from build123d import *

# Parameters (mm, degrees)
SKETCH_1_R      = 4
SKETCH_1_R_2    = 1.55
EXTRUDE_1_DEPTH = 4
SKETCH_2_R      = 10
SKETCH_2_R_2    = 1.55
EXTRUDE_2_DEPTH = 3


with BuildPart() as part:
    # 草图1 → 凸台-拉伸1 (new body)
    with BuildSketch(Plane(origin=(0, 0, 0), x_dir=(1, 0, 0), z_dir=(0, 1, 0))):
        with Locations(Location((0, 0, 0), (0, 0, 270))):
            Circle(SKETCH_1_R)
        with Locations(Location((0, 0, 0), (0, 0, 270))):
            Circle(SKETCH_1_R_2, mode=Mode.SUBTRACT)
    extrude(amount=EXTRUDE_1_DEPTH)

    # 草图2 → 凸台-拉伸2 (add)
    with BuildSketch(Plane(origin=(0, 4, 0), x_dir=(1, 0, 0), z_dir=(0, 1, 0))):
        with Locations(Location((0, 0, 0), (0, 0, 270))):
            Circle(SKETCH_2_R)
        with Locations(Location((0, 0, 0), (0, 0, 270))):
            Circle(SKETCH_2_R_2, mode=Mode.SUBTRACT)
        with Locations(Location((0, 7, 0), (0, 0, 270))):
            Circle(SKETCH_2_R_2, mode=Mode.SUBTRACT)
        with Locations(Location((7, 0, 0), (0, 0, 270))):
            Circle(SKETCH_2_R_2, mode=Mode.SUBTRACT)
        with Locations(Location((0, -7, 0), (0, 0, 270))):
            Circle(SKETCH_2_R_2, mode=Mode.SUBTRACT)
        with Locations(Location((-7, 0, 0), (0, 0, 270))):
            Circle(SKETCH_2_R_2, mode=Mode.SUBTRACT)
    extrude(amount=EXTRUDE_2_DEPTH)


solid = part.part
Can you work these out from the model? Positions are in its coordinate system, mm. A direction names the side the tool comes from. Give positions to 0.01 mm unless a question says otherwise; leave off trailing zeros. Order: outer loops, then holes, each group sorted by start corner. A loop starts at its lowest first (then second) coordinate and runs counter-clockwise, first axis right, second up. Notation, with made-up numbers: (-14.5, 55) - (-4.5, 55) arc R6 cw to (-4.5, 65) - close; hole circle Ø8 at (72, 77.25). An arc over 180 degrees is marked (long way). Write each question's results on one line, items separated by ' | '.
1) Suppose I cut it at A-A, the plane z = 0. Write out the boundary of the cut face in (x, y), then the cut area to 3 significant figures.
Final values:
outline: (-10, 4) - (-8.55, 4) - (-8.55, 7) - (-10, 7) - close; (-5.45, 4) - (-4, 4) - (-4, 0) - (-1.55, 0) - (-1.55, 7) - (-5.45, 7) - close; (1.55, 0) - (4, 0) - (4, 4) - (5.45, 4) - (5.45, 7) - (1.55, 7) - close; (8.55, 4) - (10, 4) - (10, 7) - (8.55, 7) - close | area: 51.7 mm^2
2) Suppose I cut it at C-C, the plane y = 5.5. Write out the boundary of the cut face in (x, z).
Final values:
outline: circle Ø20 at (0, 0); hole circle Ø3.1 at (-7, 0); hole circle Ø3.1 at (0, -7); hole circle Ø3.1 at (0, 0); hole circle Ø3.1 at (0, 7); hole circle Ø3.1 at (7, 0)
3) Please list where these lines run through material, in increasing order: line 1 along X through (y, z) = (4.7, 0); line 2 along X through (y, z) = (3.25, 0); line 3 along Y through (x, z) = (-1, 9). Write a range as [from, to].
Final values:
line 1: x = [-10, -8.55], [-5.45, -1.55], [1.55, 5.45], [8.55, 10] | line 2: x = [-4, -1.55], [1.55, 4] | line 3: y = [4, 7]
4) I'm going to push flat-ended pins straight in: pin 1 Ø1 at (y, z) = (5, 6) entering from +X; pin 2 Ø3.5 at (x, z) = (0, 0) entering from -Y; pin 3 Ø2.5 at (x, z) = (0, 7) entering from -Y; pin 4 Ø2 at (y, z) = (3.5, -7) entering from +X. Where does each tip first touch, or does it pass through?
Final values:
pin 1: stops at x = 8.35 | pin 2: stops at y = 0 | pin 3: passes through | pin 4: stops at x = 7.9
5) Suppose I cut it at B-B, the plane x = 0.75. Write out the boundary of the cut face in (y, z), then the cut area to 3 significant figures.
Final values:
outline: (0, -3.93) - (4, -3.93) - (4, -5.64) - (7, -5.64) - (7, -1.36) - (0, -1.36) - close; (0, 1.36) - (7, 1.36) - (7, 5.64) - (4, 5.64) - (4, 3.93) - (0, 3.93) - close; (4, -9.97) - (7, -9.97) - (7, -8.36) - (4, -8.36) - close; (4, 8.36) - (7, 8.36) - (7, 9.97) - (4, 9.97) - close | area: 56.0 mm^2
6) On a 3-axis mill with a long thin cutter (end or side, diameter ignored), from which of +Z, -Z, +X, -X, +Y, -Y can I reach the whole of each face in a straight line? I mean faces 5 (the face through (-2, 7, 0)), 6 (the face through (0.1, 4, 4.3)). Say none if no direction works.
Final values:
face 5: +Z, -Z, +X, -X, +Y | face 6: -Y
7) If we mould it in two halves opening along Z, with no side actions, what happens to faces 1 (the face through (0, 0, 2)), 2 (the face through (5.487, 5.479, -0.336)), 3 (the face through (-8.513, 5.479, -0.336)), 4 (the face through (-3.905, 1.972, -0.867))? For each: pulls with the +Z half, pulls with the -Z half, needs draft (parallel to the pull), parting line crosses it, or undercut.
Final values:
face 1: needs draft | face 2: undercut | face 3: undercut | face 4: parting line crosses it
8) Suppose I cut it at D-D, the plane x = -7. Write out the boundary of the cut face in (y, z).
Final values:
outline: (4, -7.14) - (7, -7.14) - (7, -1.55) - (4, -1.55) - close; (4, 1.55) - (7, 1.55) - (7, 7.14) - (4, 7.14) - close
